```python
from build123d import *

# Parameters (mm, degrees)
F0_W     = 20.32
F0_H     = 20.32
F1_DEPTH = 2.54
F0_W_2   = 25.4
F0_H_2   = 25.4
F2_DEPTH = 22.86
F3_W     = 1.27
F3_H     = 2.54
F3_W_2   = 0.635
F3_H_2   = 1.27
F4_DEPTH = 1.27
F5_SIZE  = 1.26999
F6_W     = 1.27
F6_H     = 2.54
F7_DEPTH = 1.27
F8_SIZE  = 1.26999
F9_R     = 1.27


# Not quite as in the source:
# - a fillet or chamfer is up to 0.001 mm smaller than in the source, because OpenCascade refuses the exact size


with BuildPart() as f1:
    # F0 (on Top) → F1 (new body)
    with BuildSketch(Plane.XY):
        Rectangle(F0_W, F0_H)
    extrude(amount=F1_DEPTH)

    # F0 (on Top) → F2 (join)
    with BuildSketch(Plane.XY):
        Rectangle(F0_W_2, F0_H_2)
        Rectangle(F0_W, F0_H, mode=Mode.SUBTRACT)
    extrude(amount=F2_DEPTH)

    # F3 (on face) → F4 (cut)
    with BuildSketch(Plane.YZ.offset(-10.16)):
        with Locations((0, 17.78)):
            Rectangle(F3_W, F3_H)
        with Locations((0, 17.78)):
            Rectangle(F3_W_2, F3_H_2, mode=Mode.SUBTRACT)
        with Locations((0, 17.78)):
            Rectangle(F3_W_2, F3_H_2)
    extrude(amount=-F4_DEPTH, mode=Mode.SUBTRACT)

    # F5 (size 1.27 in the source; OpenCascade refuses exactly that, so slightly less here)
    f5_edges = [f1.edges().sort_by_distance(p)[0] for p in [
        (-11.43, 0, 19.05),
    ]]
    chamfer(f5_edges, length=F5_SIZE)

    # F6 (on face) → F7 (cut)
    with BuildSketch(Plane(origin=(10.16, 0, 0), x_dir=(0, -1, 0), z_dir=(-1, 0, 0))):
        with Locations((0, 17.78)):
            Rectangle(F6_W, F6_H)
    extrude(amount=-F7_DEPTH, mode=Mode.SUBTRACT)

    # F8 (size 1.27 in the source; OpenCascade refuses exactly that, so slightly less here)
    f8_edges = [f1.edges().sort_by_distance(p)[0] for p in [
        (11.43, 0, 19.05),
    ]]
    chamfer(f8_edges, length=F8_SIZE)

    # F9
    f9_edges = [f1.edges().sort_by_distance(p)[0] for p in [
        (-12.7, -12.7, 11.43),
        (12.7, -12.7, 11.43),
        (12.7, 12.7, 11.43),
        (-12.7, 12.7, 11.43),
    ]]
    fillet(f9_edges, radius=F9_R)


solid = f1.part
```
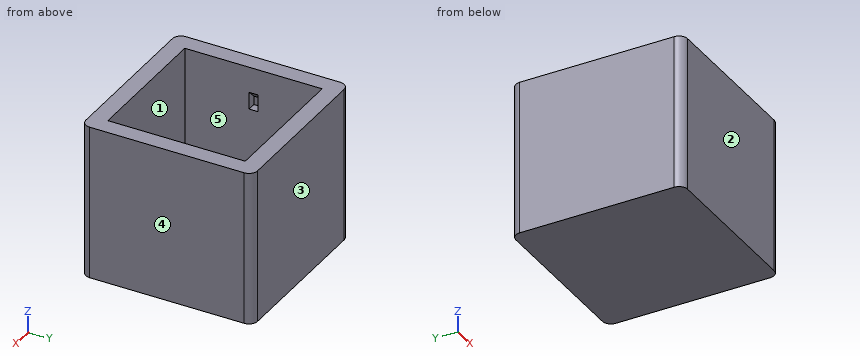
Source: CAD feature listing. Evaluate the final solid. Frame: model axes, mm. Face numbers are marked on the shaded views. A direction names the side the tool comes from. Round coordinates to 2 decimals unless told otherwise and drop trailing zeros. Loops run counter-clockwise (first coordinate to the right, second up) from the corner with the lowest first, then second, coordinate; pieces in that order, holes last. Notation, with made-up numbers: M -1.5,-21 L 25.5,-21 A16 ccw 25.5,2 Z; hole C -25,79.25 d6. An arc over 180 degrees is marked long. Use a Markdown table: item, result. Add a question column.
1. Section query B-B on x = 1.25. Return the cut outline in (y, z), then the cut area to 3 significant figures.
2. Section query A-A on z = 12. Return the cut outline in (x, y).
3. Contact query for a flat-ended pin moving along its axis: P1, Ø1.5, axis at x = -1, y = 2.5, coming from the +Z side. Output: stop coordinate, or through.
4. Line query: line 1 (Y direction, x = -2.75, z = 6.5); line 2 (Z direction, x = 1.5, y = -3). Output: solid intervals per line, ascending.
5. Reachability of the marked faces 4 and 5 from +Z, -Z, +X, -X, +Y, -Y: full face, straight path, thin tool, end or side. Return the list, or none.
6. Mould query, pull axis Y, two halves, no side actions, for the marked faces 1, 2 and 3. Classes: pulls with the +Y half, pulls with the -Y half, needs draft (parallel to the pull), parting line crosses it, or undercut.
Reported:
| question | item | result |
|---|---|---|
| 1 | outline | M -12.7,0 L 12.7,0 L 12.7,22.86 L 10.16,22.86 L 10.16,2.54 L -10.16,2.54 L -10.16,22.86 L -12.7,22.86 Z |
| 1 | area | 168 mm² |
| 2 | outline | M -12.7,-11.43 A1.27 ccw -11.43,-12.7 L 11.43,-12.7 A1.27 ccw 12.7,-11.43 L 12.7,11.43 A1.27 ccw 11.43,12.7 L -11.43,12.7 A1.27 ccw -12.7,11.43 Z; hole M -10.16,-10.16 L 10.16,-10.16 L 10.16,10.16 L -10.16,10.16 Z |
| 3 | P1 | stops at z = 2.54 |
| 4 | line 1 | y = -12.7 to -10.16, 10.16 to 12.7 |
| 4 | line 2 | z = 0 to 2.54 |
| 5 | face 4 | +Z, -Z, +X, +Y, -Y |
| 5 | face 5 | +Z |
| 6 | face 1 | undercut |
| 6 | face 2 | pulls with the -Y half |
| 6 | face 3 | pulls with the +Y half |
